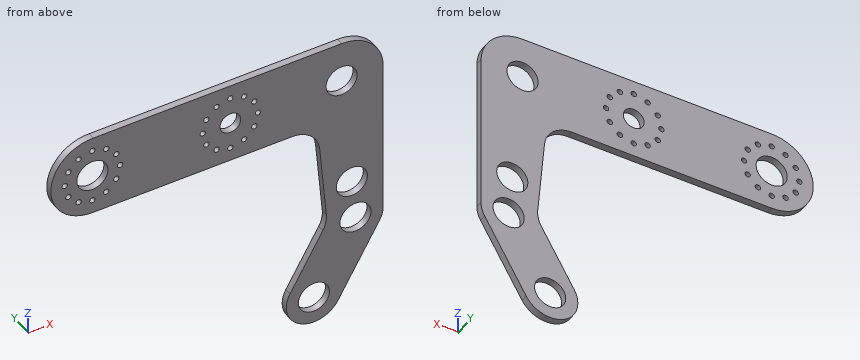
from build123d import *

# Parameters (mm, degrees)
BOSS_EXTRUDE1_OUTLINE_R   = 2.4892
BOSS_EXTRUDE1_OUTLINE_R_2 = 14.2875
BOSS_EXTRUDE1_DEPTH       = 6.35
FILLET1_R                 = 25.4
FILLET2_R                 = 25.4
SKETCH2_R                 = 9.525
SKETCH2_R_2               = 2.4892
CUT_EXTRUDE1_DEPTH        = 7.366


# Read off the part's stored shape, not the designer's step: Boss-Extrude1
with BuildPart() as part:
    # Boss-Extrude1 outline → Boss-Extrude1 (new body)
    with BuildSketch(Plane(origin=(0, 0, 0), x_dir=(1, 0, 0), z_dir=(0, 1, 0))):
        with BuildLine():
            Line((206.436572843, 38.103184831), (0, 38.103184831))
            ThreePointArc((0, 38.103184831), (-38.101592382, -0.348356423), (0.696683728, -38.096815169))
            Line((0.696683728, -38.096815169), (228.6, -38.09681517))
            ThreePointArc((228.6, -38.09681517), (255.149948273, -27.321558755), (266.68118702, -1.091110092))
            Line((266.68118702, -1.091110092), (266.729096059, 145.494235656))
            ThreePointArc((266.729096059, 145.494235656), (265.863612052, 152.068239358), (263.326141338, 158.194235572))
            Line((263.326141338, 158.194235572), (225.226141484, 224.185371425))
            ThreePointArc((225.226141484, 224.185371425), (190.529096228, 233.482416681), (181.232050972, 198.785371425))
            Line((181.232050972, 198.785371425), (215.327756353, 139.729877384))
            Line((215.327756353, 139.729877384), (206.436572843, 38.103184831))
        make_face()
        with Locations((-12.7, -21.997045256)):
            Circle(BOSS_EXTRUDE1_OUTLINE_R, mode=Mode.SUBTRACT)
        with Locations((0, -25.4)):
            Circle(BOSS_EXTRUDE1_OUTLINE_R, mode=Mode.SUBTRACT)
        with Locations((-21.997045256, -12.7)):
            Circle(BOSS_EXTRUDE1_OUTLINE_R, mode=Mode.SUBTRACT)
        with Locations((12.7, -21.997045256)):
            Circle(BOSS_EXTRUDE1_OUTLINE_R, mode=Mode.SUBTRACT)
        with Locations((21.997045256, -12.7)):
            Circle(BOSS_EXTRUDE1_OUTLINE_R, mode=Mode.SUBTRACT)
        with Locations((-25.4, 0)):
            Circle(BOSS_EXTRUDE1_OUTLINE_R, mode=Mode.SUBTRACT)
        with Locations((-21.997045256, 12.7)):
            Circle(BOSS_EXTRUDE1_OUTLINE_R, mode=Mode.SUBTRACT)
        Circle(BOSS_EXTRUDE1_OUTLINE_R_2, mode=Mode.SUBTRACT)
        with Locations((-12.7, 21.997045256)):
            Circle(BOSS_EXTRUDE1_OUTLINE_R, mode=Mode.SUBTRACT)
        with Locations((0, 25.4)):
            Circle(BOSS_EXTRUDE1_OUTLINE_R, mode=Mode.SUBTRACT)
        with Locations((25.4, 0)):
            Circle(BOSS_EXTRUDE1_OUTLINE_R, mode=Mode.SUBTRACT)
        with Locations((21.997045256, 12.7)):
            Circle(BOSS_EXTRUDE1_OUTLINE_R, mode=Mode.SUBTRACT)
        with Locations((12.7, 21.997045256)):
            Circle(BOSS_EXTRUDE1_OUTLINE_R, mode=Mode.SUBTRACT)
        with Locations((228.6, 0)):
            Circle(BOSS_EXTRUDE1_OUTLINE_R_2, mode=Mode.SUBTRACT)
        with Locations((238.001821162, 107.463307623)):
            Circle(BOSS_EXTRUDE1_OUTLINE_R_2, mode=Mode.SUBTRACT)
        with Locations((241.329096228, 145.494235656)):
            Circle(BOSS_EXTRUDE1_OUTLINE_R_2, mode=Mode.SUBTRACT)
        with Locations((203.229096228, 211.485371425)):
            Circle(BOSS_EXTRUDE1_OUTLINE_R_2, mode=Mode.SUBTRACT)
    extrude(amount=BOSS_EXTRUDE1_DEPTH)

    # Fillet1
    fillet1_edges = [part.edges().sort_by_distance(p)[0] for p in [
        (215.327756353, 3.175, -139.729877384),
    ]]
    fillet(fillet1_edges, radius=FILLET1_R)

    # Fillet2
    fillet2_edges = [part.edges().sort_by_distance(p)[0] for p in [
        (206.436572843, 3.175, -38.103184831),
    ]]
    fillet(fillet2_edges, radius=FILLET2_R)

    # Sketch2 → Cut-Extrude1 (cut)
    with BuildSketch(Plane(origin=(0, 6.35, 0), x_dir=(1, 0, 0), z_dir=(0, 1, 0))):
        with Locations(Location((126.571094876, 0, 0), (0, 0, 270))):
            Circle(SKETCH2_R)
        with Locations(Location((101.171094876, 0, 0), (0, 0, 270))):
            Circle(SKETCH2_R_2)
        with Locations(Location((104.57404962, 12.7, 0), (0, 0, 270))):
            Circle(SKETCH2_R_2)
        with Locations(Location((113.871094876, 21.997045256, 0), (0, 0, 270))):
            Circle(SKETCH2_R_2)
        with Locations(Location((126.571094876, 25.4, 0), (0, 0, 270))):
            Circle(SKETCH2_R_2)
        with Locations(Location((139.271094876, 21.997045256, 0), (0, 0, 270))):
            Circle(SKETCH2_R_2)
        with Locations(Location((148.568140132, 12.7, 0), (0, 0, 270))):
            Circle(SKETCH2_R_2)
        with Locations(Location((151.971094876, 0, 0), (0, 0, 270))):
            Circle(SKETCH2_R_2)
        with Locations(Location((148.568140132, -12.7, 0), (0, 0, 270))):
            Circle(SKETCH2_R_2)
        with Locations(Location((139.271094876, -21.997045256, 0), (0, 0, 270))):
            Circle(SKETCH2_R_2)
        with Locations(Location((126.571094876, -25.4, 0), (0, 0, 270))):
            Circle(SKETCH2_R_2)
        with Locations(Location((113.871094876, -21.997045256, 0), (0, 0, 270))):
            Circle(SKETCH2_R_2)
        with Locations(Location((104.57404962, -12.7, 0), (0, 0, 270))):
            Circle(SKETCH2_R_2)
    extrude(amount=-CUT_EXTRUDE1_DEPTH, mode=Mode.SUBTRACT)


solid = part.part
Verification items for the finished model (mm, model axes). Coordinates: 2 decimals unless noted, no trailing zeros. Order: outer loops, then holes, each group sorted by start corner. A loop starts at its lowest first (then second) coordinate and runs counter-clockwise, first axis right, second up. Notation, with made-up numbers: (35.5, 86.5) -> (50.5, 86.5) arc R13 ccw to (50.5, 108.5) -> close; hole circle Ø5 at (-39.75, 58). An arc over 180 degrees is marked (long way). Use CSV: the item, a comma, the result in double quotes. Start each with the question number.
Q1. Section check A-A, the plane z = -219. Record the cut outline in (x, y).
Q2. Depth check by flat-ended pin: P1, Ø2, axis at y = 5.5, z = -32, coming from the -X side; P2, Ø2, axis at x = 53, y = 5, coming from the -Z side; P3, Ø3, axis at y = 5.5, z = -131.5, coming from the +X side (3 decimals). Enter the tip coordinate at first touch or a pass-through.
Q3. Section check B-B, the plane z = -151. Record the cut outline in (x, y), and give its area (3 significant figures).
Q4. Thickness scan on line 1 along Z through (x, y) = (140.5, 1.5); line 2 along X through (y, z) = (5, 25.4); line 3 along Z through (x, y) = (150.5, 3). Record the ranges inside material, lowest first.
Q5. Section check C-C, the plane y = 1.5. Give the number of separate pieces and of enclosed holes in the cut face, and give its area (3 significant figures).
Returned:
1,outline,"(178.97, 0) -> (191.08, 0) -> (191.08, 6.35) -> (178.97, 6.35) -> close; (215.38, 0) -> (228.22, 0) -> (228.22, 6.35) -> (215.38, 6.35) -> close"
2,P1,"stops at x = -22.16"
2,P2,"stops at z = -38.1"
2,P3,"stops at x = 266.725"
3,outline,"(208.82, 0) -> (228.15, 0) -> (228.15, 6.35) -> (208.82, 6.35) -> close; (254.51, 0) -> (266.13, 0) -> (266.13, 6.35) -> (254.51, 6.35) -> close"
3,area,"196 mm^2"
4,line 1,"z = -38.1 to -24.16, -19.83 to 19.83, 24.16 to 38.1"
4,line 2,"x = -28.4 to -2.49, 2.49 to 124.08, 129.06 to 256.99"
4,line 3,"z = -38.1 to -14.27, -11.13 to -2.01, 2.01 to 11.13, 14.27 to 38.1"
5,separate pieces,"1"
5,enclosed holes,"30"
5,area,"29,300 mm^2"
